Model file for the job. Use its own axes, mm. Round coordinates to 2 decimals unless told otherwise and drop trailing zeros. Loops run counter-clockwise (first coordinate to the right, second up) from the corner with the lowest first, then second, coordinate; pieces in that order, holes last. Notation, with made-up numbers: M 76,-28.75 L 117,-28.75 A19 cw 117,-23.75 Z; hole C 11,74 d10. An arc over 180 degrees is marked long. Answer in a Markdown table with one row per item.
Autodesk Inventor part; units mm, degrees
ref_plane "YZ Plane" through (0, 0, 0) normal (1, 0, 0) x (0, 1, 0)
ref_plane "XZ Plane" through (0, 0, 0) normal (0, 1, 0) x (-1, 0, 0)
ref_plane "XY Plane" through (0, 0, 0) normal (0, 0, 1) x (1, 0, 0)
sketch "Sketch1" plane through (0, 0, 0) normal (1, 0, 0) x (0, 1, 0)
  line L0 (-7, 22) -> (-7, -22)
  line L1 (-7, -22) -> (7, -22)
  line L2 (7, -22) -> (7, 22)
  line L3 (7, 22) -> (-7, 22)
  line L4 (-7, 22) -> (7, -22) construction
  line L5 (-7, -22) -> (7, 22) construction
  point P0 (0, 0)
  dimension "d0" = 44
  dimension "d1" = 14
extrude "Extrusion1" add sketch "Sketch1" along normal blind 3
sketch "Sketch2" plane through (3, 0, 0) normal (1, 0, 0) x (0, 0, -1)
  line L0 (0, 0) -> (16.154, 0)
  circle A0 centre (16.154, 0) radius 1.5
  dimension "d4" = 16.154
  dimension "d5" = 3
extrude "Extrusion2" cut sketch "Sketch2" against normal blind 3
thread "Thread1"
mirror "Mirror1" about plane through (0, 0, 0) normal (0, 0, 1) of "Extrusion2"
fillet "Fillet1" radius 0.6 12 edges at (3, -7, 0) (0, -7, 0) (1.5, -7, -22) (3, 0, -22) (0, 0, -22) (1.5, 7, -22) (3, 7, 0) (0, 7, 0) (1.5, 7, 22) (3, 0, 22) (1.5, -7, 22) (0, 0, 22)
properties part number "Clamp Plate"
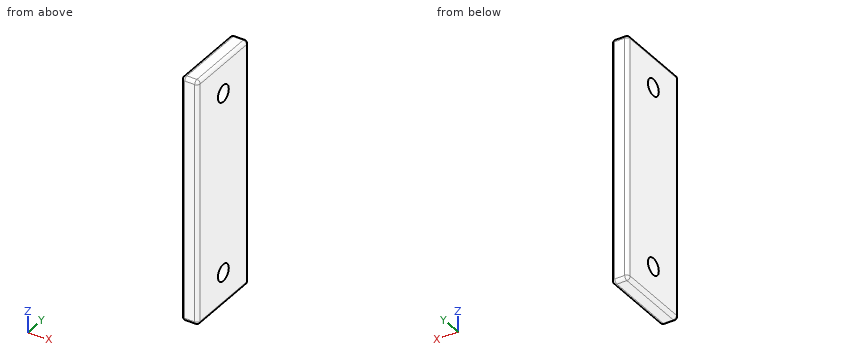
1. Saw through at B-B (x = 1.7). Write the cut outline in (y, z), and give its area (3 significant figures).
Verdict:
| item | result |
|---|---|
| outline | M -7,-21.4 A0.6 ccw -6.4,-22 L 6.4,-22 A0.6 ccw 7,-21.4 L 7,21.4 A0.6 ccw 6.4,22 L -6.4,22 A0.6 ccw -7,21.4 Z; hole C 0,-16.15 d3; hole C 0,16.15 d3 |
| area | 602 mm² |
2. Saw through at A-A (y = 0). Write the cut outline in (x, z).
Verdict:
| item | result |
|---|---|
| outline | M 0,-21.4 A0.6 ccw 0.6,-22 L 2.4,-22 A0.6 ccw 3,-21.4 L 3,-17.65 L 0,-17.65 Z; M 0,-14.65 L 3,-14.65 L 3,14.65 L 0,14.65 Z; M 0,17.65 L 3,17.65 L 3,21.4 A0.6 ccw 2.4,22 L 0.6,22 A0.6 ccw 0,21.4 Z |
3. Wall check: probe 1 along Z at (x, y) = (1.35, 0); probe 2 along Z at (x, y) = (2.7, -1); probe 3 along Z at (x, y) = (2.45, 3.25). Give the ranges that are in metal, low to high.
Verdict:
| item | result |
|---|---|
| probe 1 | z = -22 to -17.65, -14.65 to 14.65, 17.65 to 22 |
| probe 2 | z = -21.92 to -17.27, -15.04 to 15.04, 17.27 to 21.92 |
| probe 3 | z = -22 to 22 |
